from build123d import *

# Parameters (mm, degrees)
SKETCH1_R              = 2.38125
BOSS_EXTRUDE1_DEPTH    = 19.685
SKETCH2_W              = 15.5956
SKETCH2_H              = 12.7
CUT_EXTRUDE1_DEPTH     = 65.401648659
FILLET1_R              = 6.35
SKETCH3_R              = 2.38125
SKETCH3_W              = 25.4
SKETCH3_H              = 12.7
CUT_EXTRUDE2_DEPTH     = 65.40164869
FILLET2_R              = 3.175
CUT_EXTRUDE5_OUTLINE_R = 4.7625
CUT_EXTRUDE5_DEPTH     = 2.149867926


with BuildPart() as part:
    # Sketch1 → Boss-Extrude1 (new body)
    with BuildSketch(Plane(origin=(0, 0, 0), x_dir=(1, 0, 0), z_dir=(0, 1, 0))):
        with BuildLine():
            Line((0, 5.08), (24.690664344, 21.076673302))
            ThreePointArc((24.690664344, 21.076673302), (28.575, 22.225), (32.459335656, 21.076673302))
            Line((32.459335656, 21.076673302), (57.15, 5.08))
            Line((57.15, 5.08), (57.15, 0))
            Line((57.15, 0), (0, 0))
            Line((0, 0), (0, 5.08))
        make_face()
        with Locations(Location((28.575, 15.08125, 0), (0, 0, 270))):
            Circle(SKETCH1_R, mode=Mode.SUBTRACT)
    extrude(amount=-BOSS_EXTRUDE1_DEPTH)

    # Sketch2 → Cut-Extrude1 (cut, through all)
    with BuildSketch(Plane(origin=(57.15, 0, 0), x_dir=(0, 0, -1), z_dir=(1, 0, 0))):
        with Locations((14.4272, -9.8425)):
            Rectangle(SKETCH2_W, SKETCH2_H)
    extrude(amount=-CUT_EXTRUDE1_DEPTH, mode=Mode.SUBTRACT)

    # Fillet1
    fillet1_edges = [part.edges().sort_by_distance(p)[0] for p in [
        (28.575, -16.1925, -6.6294),
        (28.575, -3.4925, -6.6294),
    ]]
    fillet(fillet1_edges, radius=FILLET1_R - 0.0001)  # a hair under: the kernel refuses the full size

    # Sketch3 → Cut-Extrude2 (cut, through all)
    with BuildSketch(Plane.XY):
        with Locations((9.525, -9.8425)):
            Circle(SKETCH3_R)
        with Locations((47.625, -9.8425)):
            Circle(SKETCH3_R)
        with Locations((28.575, -9.8425)):
            Rectangle(SKETCH3_W, SKETCH3_H)
    extrude(amount=-CUT_EXTRUDE2_DEPTH, mode=Mode.SUBTRACT)

    # Fillet2
    fillet2_edges = [part.edges().sort_by_distance(p)[0] for p in [
        (41.275, -3.4925, -6.48965),
        (15.875, -16.1925, -6.48965),
        (41.275, -16.1925, -6.48965),
        (15.875, -3.4925, -6.48965),
    ]]
    fillet(fillet2_edges, radius=FILLET2_R)

    # Cut-Extrude5: read off the stored shape, not the designer's step
    # Cut-Extrude5 outline → Cut-Extrude5 (cut)
    with BuildSketch(Plane(origin=(0, 0, -6.6294), x_dir=(-1, 0, 0), z_dir=(0, 0, -1))):
        with Locations((-47.625, -9.8425)):
            Circle(CUT_EXTRUDE5_OUTLINE_R)
        with Locations((-9.525, -9.8425)):
            Circle(CUT_EXTRUDE5_OUTLINE_R)
    extrude(amount=CUT_EXTRUDE5_DEPTH, mode=Mode.SUBTRACT)


solid = part.part
Geometry: final body of the model. Coordinates: model frame, mm. A direction names the side the tool comes from. Coordinates: 2 decimals unless noted, no trailing zeros. Order: outer loops, then holes, each group sorted by start corner. A loop starts at its lowest first (then second) coordinate and runs counter-clockwise, first axis right, second up.
(1) Section query A-A (x = 24). Return the cut outline in (y, z) (1 decimal).
(2) Section query B-B (z = -3.75). State how many separate pieces and enclosed holes the cut face has, plus the area to 3 significant figures.
(3) Section query D-D (z = -15.75). Return the cut outline in (x, y) (1 decimal), plus the area to 3 significant figures.
(4) Material intervals for probe 1 along X at (y, z) = (-12.5, -4.5) (3 decimals); probe 2 along Y at (x, z) = (25, -3.25) (1 decimal); probe 3 along Z at (x, y) = (5.5, -13), sorted ascending.
(5) First-contact query: pin 1 (1 mm diameter, centred on x = 7, y = -8, fed in from -Z); pin 2 (4 mm diameter, centred on x = 28.58, z = -15.08, fed in from -Y); pin 3 (7.5 mm diameter, centred on x = 7, y = -11.5, fed in from -Z); pin 4 (3 mm diameter, centred on x = 10.5, y = -3.5, fed in from -Z). Flat tips, straight axial feed; report the tip coordinate or a pass-through.
(6) Draft query along Y for faces 5 (the face through (46.31, -15.08, -9.39)), 6 (the face through (9.43, -3.14, -11.19)), 7 (the face through (15.875, -10, -4)), 8 (the face through (29, 0, -9)). Return one class per face: pulls with the +Y half, pulls with the -Y half, needs draft (parallel to the pull), parting line crosses it, or undercut.
(7) Access query for faces 1 (the face through (12.46, -4.68, -9.28)), 2 (the face through (29, -3, 0)), 3 (the face through (39.95, -15.6, -5.14)), 4 (the face through (29, -16.192, -11)). Directions: +Z, -Z, +X, -X, +Y, -Y. A direction counts if a zero-diameter tool reaches every point of the face in a straight line with its end or side. Return the directions, or none.
Solution:
1. outline: (-19.7, -20.6) - (-16.2, -20.6) - (-16.2, 0) - (-19.7, 0) - close; (-3.5, -20.6) - (0, -20.6) - (0, 0) - (-3.5, 0) - close
2. separate pieces: 1
2. enclosed holes: 3
2. area: 775 mm2
3. outline: (16.5, -19.7) - (26.3, -19.7) - (26.3, -16.2) - (16.5, -16.2) - close; (16.5, -3.5) - (26.3, -3.5) - (26.3, 0) - (16.5, 0) - close; (30.9, -19.7) - (40.7, -19.7) - (40.7, -16.2) - (30.9, -16.2) - close; (30.9, -3.5) - (40.7, -3.5) - (40.7, 0) - (30.9, 0) - close
3. area: 137 mm2
4. probe 1: x = 0 to 15.875, 41.275 to 57.15
4. probe 2: y = -19.7 to -16.2, -3.5 to 0
4. probe 3: z = -7.47 to 0
5. pin 1: stops at z = -6.63
5. pin 2: passes through
5. pin 3: stops at z = -9.65
5. pin 4: stops at z = -12.85
6. face 5: undercut
6. face 6: needs draft
6. face 7: undercut
6. face 8: pulls with the +Y half
7. face 1: -Z, +X, -X
7. face 2: +Z, +X, -X, +Y, -Y
7. face 3: +Z, -Z
7. face 4: -Z
